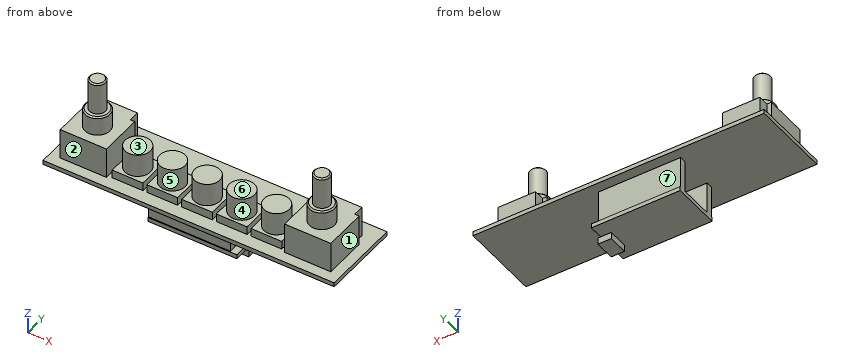
```python
from build123d import *

# Parameters (mm, degrees)
F0_W      = 11.5
F0_H      = 11.5
F1_DEPTH  = 4.7
F0_W_2    = 109
F0_H_2    = 30
F2_DEPTH  = 1.6
F3_R      = 4.75
F4_DEPTH  = 8.6
F5_W      = 14
F5_H      = 4
F6_DEPTH  = 11.5
F7_R      = 4.7
F8_DEPTH  = 7.2
F9_R      = 3
F10_DEPTH = 12
F11_SIZE  = 0.5
F12_W     = 1.5
F12_H     = 2.5
F12_W_2   = 11.5
F12_W_3   = 2.65
F12_W_4   = 0.55
F12_W_5   = 30.7
F13_DEPTH = 12
F14_W     = 30.7
F14_H     = 2.5
F15_DEPTH = 1.6
F16_W     = 4
F16_H     = 7.5
F16_W_2   = 1
F17_DEPTH = 2.5


with BuildPart() as f1:
    # F0 (on Top) → F1 (new body)
    with BuildSketch(Plane.XY):
        with Locations((-26, -4.45)):
            Rectangle(F0_W, F0_H)
    extrude(amount=F1_DEPTH)



with BuildPart() as f1b:
    # F0 (on Top) → F1, piece 2 (new body)
    with BuildSketch(Plane.XY):
        with Locations((-13, -4.45)):
            Rectangle(F0_W, F0_H)
    extrude(amount=F1_DEPTH)


with BuildPart() as f1c:
    # F0 (on Top) → F1, piece 3 (new body)
    with BuildSketch(Plane.XY):
        with Locations((13, -4.45)):
            Rectangle(F0_W, F0_H)
    extrude(amount=F1_DEPTH)


with BuildPart() as f1d:
    # F0 (on Top) → F1, piece 4 (new body)
    with BuildSketch(Plane.XY):
        with Locations((26, -4.45)):
            Rectangle(F0_W, F0_H)
    extrude(amount=F1_DEPTH)


with BuildPart() as f1e:
    # F0 (on Top) → F1, piece 5 (new body)
    with BuildSketch(Plane.XY):
        with Locations((0, -4.45)):
            Rectangle(F0_W, F0_H)
    extrude(amount=F1_DEPTH)


with BuildPart() as f1_1:
    add(f1.part)

    add(f1b.part)  # F2 merges F1b

    add(f1c.part)  # F2 merges F1c

    add(f1d.part)  # F2 merges F1d

    add(f1e.part)  # F2 merges F1e
    # F0 (on Top) → F2 (join)
    with BuildSketch(Plane.XY):
        Rectangle(F0_W_2, F0_H_2)
        with Locations((-26, -4.45)):
            Rectangle(F0_W, F0_H, mode=Mode.SUBTRACT)
        with Locations((-13, -4.45)):
            Rectangle(F0_W, F0_H, mode=Mode.SUBTRACT)
        with Locations((0, -4.45)):
            Rectangle(F0_W, F0_H, mode=Mode.SUBTRACT)
        with Locations((13, -4.45)):
            Rectangle(F0_W, F0_H, mode=Mode.SUBTRACT)
        with Locations((26, -4.45)):
            Rectangle(F0_W, F0_H, mode=Mode.SUBTRACT)
    extrude(amount=F2_DEPTH)

    # F3 (on face) → F4 (join)
    with BuildSketch(Plane.XY.offset(4.7)):
        with Locations((-26, -4.45)):
            Circle(F3_R)
        with Locations((-13, -4.45)):
            Circle(F3_R)
        with Locations((0, -4.45)):
            Circle(F3_R)
        with Locations((13, -4.45)):
            Circle(F3_R)
        with Locations((26, -4.45)):
            Circle(F3_R)
    extrude(amount=F4_DEPTH)

    # F5 (on face) → F6 (join)
    with BuildSketch(Plane.XY.offset(1.6)):
        Polygon((-50.65, -11.05), (-33.35, -11.05), (-33.35, 5.05), (-35, 5.05), (-49, 5.05), (-50.65, 5.05), align=None)
        with Locations((-42, 7.05)):
            Rectangle(F5_W, F5_H)
        with Locations((42, 7.05)):
            Rectangle(F5_W, F5_H)
        Polygon((33.35, -11.05), (50.65, -11.05), (50.65, 5.05), (49, 5.05), (35, 5.05), (33.35, 5.05), align=None)
    extrude(amount=F6_DEPTH)

    # F7 (on face) → F8 (join)
    with BuildSketch(Plane.XY.offset(13.1)):
        with Locations((-42, -3)):
            Circle(F7_R)
        with Locations((42, -3)):
            Circle(F7_R)
    extrude(amount=F8_DEPTH)

    # F9 (on face) → F10 (join)
    with BuildSketch(Plane.XY.offset(20.3)):
        with Locations((-42, -3)):
            Circle(F9_R)
        with Locations((42, -3)):
            Circle(F9_R)
    extrude(amount=F10_DEPTH)

    # F11
    f11_edges = [f1_1.edges().sort_by_distance(p)[0] for p in [
        (-46.7, -3, 20.3),
        (37.3, -3, 20.3),
        (-45, -3, 32.3),
        (39, -3, 32.3),
    ]]
    chamfer(f11_edges, length=F11_SIZE)

    # F12 (on face) → F13 (join)
    with BuildSketch(Plane.XY):
        with Locations((-19.5, -5)):
            Rectangle(F12_W, F12_H)
        with Locations((-13, -5)):
            Rectangle(F12_W_2, F12_H)
        with Locations((-6.5, -5)):
            Rectangle(F12_W, F12_H)
        with Locations((0, -5)):
            Rectangle(F12_W_2, F12_H)
        with Locations((6.5, -5)):
            Rectangle(F12_W, F12_H)
        with Locations((8.575, -5)):
            Rectangle(F12_W_3, F12_H)
        with Locations((-20.525, -5)):
            Rectangle(F12_W_4, F12_H)
        with Locations((-5.45, 10)):
            Rectangle(F12_W_5, F12_H)
    extrude(amount=-F13_DEPTH)

    # F14 (on face) → F15 (join)
    with BuildSketch(Plane(origin=(0, 0, -12), x_dir=(1, 0, 0), z_dir=(0, 0, -1))):
        Polygon((-20.8, -11.25), (-20.8, -11.55), (12.5, -11.55), (12.5, 6.55), (-20.8, 6.55), (-20.8, -8.75), (9.9, -8.75), (9.9, -11.25), align=None)
        with Locations((-5.45, -10)):
            Rectangle(F14_W, F14_H)
    extrude(amount=F15_DEPTH)

    # F16 (on face) → F17 (join)
    with BuildSketch(Plane(origin=(0, 0, -13.6), x_dir=(1, 0, 0), z_dir=(0, 0, -1))):
        with Locations((10.5, -2.5)):
            Rectangle(F16_W, F16_H)
        with Locations((13, -2.5)):
            Rectangle(F16_W_2, F16_H)
    extrude(amount=F17_DEPTH)


solid = f1_1.part
```
Input: part model. Units: mm. Frame: model coordinates. Face numbers are marked on the shaded views. A direction names the side the tool comes from. Give positions to 0.01 mm unless a question says otherwise; leave off trailing zeros. Order: outer loops, then holes, each group sorted by start corner. A loop starts at its lowest first (then second) coordinate and runs counter-clockwise, first axis right, second up.
1. Line query: probe 1 along Y at (x, z) = (-5, -10); probe 2 along Z at (x, y) = (-5.5, 3); probe 3 along Z at (x, y) = (27, 0.75). Output: solid intervals per line, ascending.
Computed:
probe 1: y = -6.25 to -3.75, 8.75 to 11.25
probe 2: z = -13.6 to -12, 0 to 1.6
probe 3: z = 0 to 4.7
2. Cut plane A-A (z = -11). Return loops of the section in (x, y), and give its area (4 significant figures).
Computed:
outline: (-20.8, -6.25) - (9.9, -6.25) - (9.9, -3.75) - (-20.8, -3.75) - close; (-20.8, 8.75) - (9.9, 8.75) - (9.9, 11.25) - (-20.8, 11.25) - close
area: 153.5 mm2
3. Cut plane C-C (x = 26). Return loops of the section in (y, z), and give its area (3 significant figures).
Computed:
outline: (-15, 0) - (15, 0) - (15, 1.6) - (1.3, 1.6) - (1.3, 4.7) - (0.3, 4.7) - (0.3, 13.3) - (-9.2, 13.3) - (-9.2, 4.7) - (-10.2, 4.7) - (-10.2, 1.6) - (-15, 1.6) - close
area: 165 mm2
4. Cut plane B-B (x = 0). Return loops of the section in (y, z), and give its area (3 significant figures).
Computed:
outline: (-15, 0) - (-6.25, 0) - (-6.25, -12) - (-6.55, -12) - (-6.55, -13.6) - (11.55, -13.6) - (11.55, -12) - (11.25, -12) - (11.25, 0) - (15, 0) - (15, 1.6) - (1.3, 1.6) - (1.3, 4.7) - (0.3, 4.7) - (0.3, 13.3) - (-9.2, 13.3) - (-9.2, 4.7) - (-10.2, 4.7) - (-10.2, 1.6) - (-15, 1.6) - close; hole (-3.75, -12) - (8.75, -12) - (8.75, 0) - (-3.75, 0) - close
area: 254 mm2
5. Draft query along Z for the marked faces 5, 6 and 7. Return one class per face: released by +Z, released by -Z, zero draft, split by the parting line, or undercut.
Computed:
face 5: zero draft
face 6: released by +Z
face 7: undercut
6. Cut plane D-D (z = 27). Return loops of the section in (x, y).
Computed:
outline: circle Ø6 at (-42, -3); circle Ø6 at (42, -3)
7. Set-up query: the marked faces 1, 2, 3 and 4. Return all of +Z, -Z, +X, -X, +Y, -Y with unobstructed straight access to the full face (end or side cutting, diameter ignored); none if empty.
Computed:
face 1: +Z, +X, +Y, -Y
face 2: +Z, +X, -X, -Y
face 3: +Z, +Y, -Y
face 4: +Z
8. Pin query (flat end, axial travel): pin 1 Ø8 at (x, y) = (38, -3.5) entering from -Z; pin 2 Ø1.3 at (x, z) = (-11.5, -12.5) entering from +Y; pin 3 Ø1.6 at (y, z) = (-5.5, 3) entering from +X. Return the tip coordinate at first contact, or that it passes through.
Computed:
pin 1: stops at z = 0
pin 2: stops at y = 11.55
pin 3: stops at x = 50.65
